Part model, mm, in its own coordinate system. Give positions to 0.01 mm unless a question says otherwise; leave off trailing zeros. Write each loop counter-clockwise with the first axis right and the second up, starting at its lowest first coordinate (ties: lowest second). Pieces come first, ordered by that corner, then holes. Notation, with made-up numbers: M 15.5,-31.5 L 37.5,-31.5 A17 ccw 37.5,-18.5 Z; hole C -40,62.5 d5. An arc over 180 degrees is marked long. Answer as CSV lines item,"result". Start each with the question number.
Item 1: Pin check, flat tips, straight feed: pin 1 (3 mm diameter, centred on x = 11.03, z = 19.45, fed in from +Y); pin 2 (5 mm diameter, centred on y = 4.5, z = 8.5, fed in from -X); pin 3 (3.5 mm diameter, centred on x = 57.13, z = 65.55, fed in from -Y); pin 4 (1 mm diameter, centred on x = 44.5, y = 1, fed in from -Z). Stop position of each tip, or through.
Item 2: Two-plate mould, pull along Z, no slides. Class faces 1 (the cylindrical face through (33.14, 3.25, 0.01)), 2 (the cylindrical face through (35.01, 3.25, 84.99)), 3 (the cylindrical face through (12.228, 3.122, 65.054)): +Z half, -Z half, draft (parallel to the pull), parting line (faces both ways), or undercut.
Item 3: Band-saw the part on C-C, the plane x = 42. List the corners of the cut face in (y, z).
Item 4: Band-saw the part on B-B, the plane z = 45.5. List the corners of the cut face in (x, y), then the cut area to 3 significant figures.
Item 5: Band-saw the part on A-A, the plane y = 3.75. List the corners of the cut face in (x, z).
Item 6: Wall check: L1, parallel to Z at x = 56, y = 0.75; L2, parallel to Z at x = 57, y = 2; L3, parallel to X at y = 6, z = 20.5. Give the ranges that are in metal, low to high. Write a range as from..to.
Autodesk Inventor part; units mm, degrees
ref_plane "YZ Plane" through (0, 0, 0) normal (1, 0, 0) x (0, 1, 0)
ref_plane "XZ Plane" through (0, 0, 0) normal (0, 1, 0) x (-1, 0, 0)
ref_plane "XY Plane" through (0, 0, 0) normal (0, 0, 1) x (1, 0, 0)
sketch "Sketch1" plane through (0, 0, 0) normal (0, 0, 1) x (1, 0, 0)
  arc A0 (76.5789, 0) -> (-8.4211, 0) centre (34.0789, -102.0754) ccw
  line L0 (-8.4211, 0) -> (76.5789, 0)
  point P0 (0, 0)
  dimension "d0" = 85
extrude "Extrusion1" add sketch "Sketch1" along normal blind 85
sketch "Sketch2" plane through (-8.4211, 0, 0) normal (0, -1, 0) x (1, 0, 0)
  circle A0 centre (7.5, 77.5) radius 0.75
  circle A1 centre (7.5, 7.5) radius 0.75
  circle A2 centre (77.5, 77.5) radius 0.75
  circle A3 centre (77.5, 7.5) radius 0.75
  line L0 (0, 85) -> (85, 85)
  line L1 (0, 0) -> (85, 0)
  line L2 (85, 0) -> (85, 85)
  point P0 (8.4211, 0)
  point P1 (36.7967, 13.095)
  dimension "d3" = 1.5
  dimension "d4" = 1.5
  dimension "d5" = 1.5
  dimension "d6" = 1.5
  dimension "d7" = 70
  dimension "d8" = 7.5
  dimension "d9" = 7.5
  dimension "d10" = 70
  dimension "d11" = 70
  dimension "d12" = 70
  dimension "d13" = 7.5
  dimension "d14" = 7.5
extrude "Extrusion2" cut sketch "Sketch2" against normal blind 85
sketch "Sketch3" plane through (-8.4211, 0, 0) normal (0, -1, 0) x (1, 0, 0)
  line L0 (0, 0) -> (0, 85)
  line L1 (0, 42.5) -> (85, 42.5)
  line L2 (85, 0) -> (85, 85)
  line L3 (0, 85) -> (85, 85)
  line L4 (42.5, 85) -> (42.5, 0)
  circle A0 centre (42.5, 42.5) radius 42.5
  line L5 (0, 0) -> (85, 0)
  line L6 (85, 85) -> (0, 85)
  line L7 (0, 85) -> (0, 0)
  line L8 (0, 0) -> (85, 0)
  line L9 (85, 0) -> (85, 85)
  point P0 (8.4211, 0)
  dimension "d17" = 42.5
extrude "Extrusion3" cut sketch "Sketch3" against normal blind 100 contours L0 A0 L5 | L0 L3 A0 | A0 L2 L5 | L3 L2 A0
sketch "Sketch4" plane through (34.0789, 0, 42.5) normal (0, -1, 0) x (1, 0, 0)
  arc A0 (-42.5, 0) -> (42.5, 0) centre (0, 0) ccw
  line L0 (0, 0) -> (42.5, 0) construction
  line L1 (30.052, 30.052) -> (-30.052, 30.052)
  line L2 (-30.052, 30.052) -> (-30.052, -30.052)
  line L3 (-30.052, -30.052) -> (30.052, -30.052)
  line L4 (30.052, -30.052) -> (30.052, 30.052)
  circle A1 centre (-23.052, 23.052) radius 1.3
  circle A2 centre (23.052, 23.052) radius 1.3
  circle A3 centre (-23.052, -23.052) radius 1.3
  circle A4 centre (23.052, -23.052) radius 1.3
  point P0 (-34.0789, -42.5)
  dimension "d21" = 2.6
  dimension "d22" = 2.6
  dimension "d23" = 2.6
  dimension "d24" = 2.6
  dimension "d29" = 7
  dimension "d30" = 7
  dimension "d31" = 7
  dimension "d32" = 7
  dimension "d33" = 7
  dimension "d34" = 7
  dimension "d35" = 7
  dimension "d36" = 7
extrude "Extrusion4" cut sketch "Sketch4" against normal blind 100 contours A1 | A2 | A3 | A4
properties part number "TopHead"
Output:
1,pin 1,"y = 6.37"
1,pin 2,"x = 5.55"
1,pin 3,"y = 0"
1,pin 4,"z = 1.17"
2,face 1,"-Z half"
2,face 2,"+Z half"
2,face 3,"undercut"
3,outline,"M 0,0.74 L 8.21,0.74 L 8.21,84.26 L 0,84.26 Z"
4,outline,"M -8.32,0 L 76.47,0 L 76.47,0.04 A110.57 ccw -8.32,0.04 Z"
4,area,"485 mm²"
5,outline,"M 2.04,14.58 A42.5 ccw 66.12,14.58 L 66.12,70.42 A42.5 ccw 2.04,70.42 Z; hole C 11.03,19.45 d2.6; hole C 11.03,65.55 d2.6; hole C 57.13,19.45 d2.6; hole C 57.13,65.55 d2.6"
6,L1,"6.09..18.81, 20.09..64.91, 66.19..78.91"
6,L2,"6.71..18.15, 20.74..64.26, 66.85..78.29"
6,L3,"11.79..56.37"
